CAD build for the part. Positions are in the model's coordinates, mm. A direction names the side the tool comes from. Coordinates: 2 decimals unless noted, no trailing zeros. Order: outer loops, then holes, each group sorted by start corner. A loop starts at its lowest first (then second) coordinate and runs counter-clockwise, first axis right, second up.
from build123d import *

# Parameters (mm, degrees)
F1_W      = 111.125
F1_H      = 63.0682
F2_DEPTH  = 1.5875
F3_W      = 111.125
F3_H      = 63.0682
F3_R      = 1.190625
F4_DEPTH  = 12.7
F5_R      = 2.38125
F7_DEPTH  = 1.5875
F9_R      = 1.5875
F10_DEPTH = 1.5875
F11_R     = 2.38125
F12_DEPTH = 3.175
F13_R     = 1.190625
F14_DEPTH = 4.7635
F15_R     = 1.190625
F16_DEPTH = 14.2885


with BuildPart() as f2:
    # F1 (on Top) → F2 (new body)
    with BuildSketch(Plane.XY):
        Rectangle(F1_W, F1_H)
    extrude(amount=F2_DEPTH)

    # F3 (on face) → F4 (join)
    with BuildSketch(Plane.XY.offset(1.5875)):
        Rectangle(F3_W, F3_H)
        with Locations((-53.18125, -29.15285)):
            Circle(F3_R, mode=Mode.SUBTRACT)
        with Locations((53.18125, -29.15285)):
            Circle(F3_R, mode=Mode.SUBTRACT)
        with BuildLine():
            Line((53.18125, 26.7716), (53.975, 26.7716))
            Line((53.975, 26.7716), (53.975, -26.7716))
            Line((53.975, -26.7716), (53.18125, -26.7716))
            ThreePointArc((53.18125, -26.7716), (51.497452, -27.469052), (50.8, -29.15285))
            Line((50.8, -29.15285), (50.8, -29.9466))
            Line((50.8, -29.9466), (-50.8, -29.9466))
            Line((-50.8, -29.9466), (-50.8, -29.15285))
            ThreePointArc((-50.8, -29.15285), (-51.497452, -27.469052), (-53.18125, -26.7716))
            Line((-53.18125, -26.7716), (-53.975, -26.7716))
            Line((-53.975, -26.7716), (-53.975, 26.7716))
            Line((-53.975, 26.7716), (-53.18125, 26.7716))
            ThreePointArc((-53.18125, 26.7716), (-51.497452, 27.469052), (-50.8, 29.15285))
            Line((-50.8, 29.15285), (-50.8, 29.9466))
            Line((-50.8, 29.9466), (50.8, 29.9466))
            Line((50.8, 29.9466), (50.8, 29.15285))
            ThreePointArc((50.8, 29.15285), (51.497452, 27.469052), (53.18125, 26.7716))
        make_face(mode=Mode.SUBTRACT)
        with Locations((-53.18125, 29.15285)):
            Circle(F3_R, mode=Mode.SUBTRACT)
        with Locations((53.18125, 29.15285)):
            Circle(F3_R, mode=Mode.SUBTRACT)
    extrude(amount=F4_DEPTH)

    # F5
    f5_edges = [f2.edges().sort_by_distance(p)[0] for p in [
        (55.5625, -31.5341, 7.14375),
        (55.5625, 31.5341, 7.14375),
        (-55.5625, -31.5341, 7.14375),
        (-55.5625, 31.5341, 7.14375),
    ]]
    fillet(f5_edges, radius=F5_R)

    # F6 (on face) → F7 (cut, through all)
    with BuildSketch(Plane.YZ.offset(55.5625)):
        Polygon((-13.1445, 14.2875), (-17.5895, 14.2875), (-23.4315, 14.2875), (-23.4315, 8.763), (-17.5895, 8.763), (-13.1445, 8.763), align=None)
        Polygon((5.5245, 8.763), (13.1445, 8.763), (17.5895, 8.763), (17.5895, 14.2875), (5.5245, 14.2875), align=None)
    extrude(amount=-F7_DEPTH, mode=Mode.SUBTRACT)

    # F9 (on face) → F10 (cut, through all)
    with BuildSketch(Plane(origin=(-55.5625, 0, 0), x_dir=(0, -1, 0), z_dir=(-1, 0, 0))):
        Polygon((19.05, 14.2875), (-19.05, 14.2875), (-20.955, 3.4925), (20.955, 3.4925), align=None)
        with Locations((-23.495, 8.89)):
            Circle(F9_R)
        with Locations((23.495, 8.89)):
            Circle(F9_R)
    extrude(amount=-F10_DEPTH, mode=Mode.SUBTRACT)

    # F11 (on face) → F12 (join)
    with BuildSketch(Plane.XY.offset(1.5875)):
        with Locations((0, 12.7)):
            Circle(F11_R)
        with Locations((0, -12.7)):
            Circle(F11_R)
    extrude(amount=F12_DEPTH)

    # F13 (on face) → F14 (cut, through all)
    with BuildSketch(Plane.XY.offset(4.7625)):
        with Locations((0, 12.7)):
            Circle(F13_R)
        with Locations((0, -12.7)):
            Circle(F13_R)
    extrude(amount=-F14_DEPTH, mode=Mode.SUBTRACT)

    # F15 (on face) → F16 (cut, through all)
    with BuildSketch(Plane.XY.offset(14.2875)):
        with Locations((53.18125, 29.15285)):
            Circle(F15_R)
        with Locations((53.18125, -29.15285)):
            Circle(F15_R)
        with Locations((-53.18125, -29.15285)):
            Circle(F15_R)
        with Locations((-53.18125, 29.15285)):
            Circle(F15_R)
    extrude(amount=-F16_DEPTH, mode=Mode.SUBTRACT)


solid = f2.part
1) Two-plate mould, pull along Z, no slides. Class faces 1 (the cylindrical face through (-54.78, -24.96, 8.28)), 2 (the flat face through (1, -14, 4.762)), 3 (the flat face through (-1, 0, 0)), 4 (the flat face through (-55.562, 0, 2)): released by +Z, released by -Z, zero draft, split by the parting line, or undercut.
2) Which spindle directions (+Z, -Z, +X, -X, +Y, -Y) get a long thin tool onto all of the face, cutting with end or side? Do faces 5 (the cylindrical face through (-0.31, 15.06, 3.15)), 6 (the flat face through (0, -31, 14.288)). Say none if no direction does.
3) Slice it at B-B (y = 12.7). List the corners of the cut face in (x, z) (1 decimal), plus the area to 3 significant figures.
4) Slice it at A-A (x = 0). List the corners of the cut face in (y, z).
5) Drill centre lines: probe 1 along Y at (x, z) = (0, 2.45); probe 2 along Y at (x, z) = (26, 3); probe 3 along X at (y, z) = (25, 5.75) (1 decimal). Where is each one in solid material? Low to high.
6) Slice it at C-C (y = -6). List the corners of the cut face in (x, z) (1 decimal).
7) Pin check, flat tips, straight feed: P1, Ø4, axis at x = 8.5, y = 1, coming from the +Z side; P2, Ø3, axis at x = -53.18, y = 29.15, coming from the +Z side; P3, Ø2.5, axis at x = 0, y = -12.7, coming from the +Z side; P4, Ø0.8, axis at x = 55, z = 11, coming from the +Y side. Stop position of each tip, or through.
Worked out:
1. face 1: undercut
1. face 2: released by +Z
1. face 3: released by -Z
1. face 4: zero draft
2. face 5: +Z
2. face 6: +Z, +X, -X, +Y, -Y
3. outline: (-55.6, 0) - (-1.2, 0) - (-1.2, 4.8) - (-2.4, 4.8) - (-2.4, 1.6) - (-54, 1.6) - (-54, 3.5) - (-55.6, 3.5) - close; (1.2, 0) - (55.6, 0) - (55.6, 8.8) - (54, 8.8) - (54, 1.6) - (2.4, 1.6) - (2.4, 4.8) - (1.2, 4.8) - close
3. area: 195 mm2
4. outline: (-31.53, 0) - (-13.89, 0) - (-13.89, 4.76) - (-15.08, 4.76) - (-15.08, 1.59) - (-29.95, 1.59) - (-29.95, 14.29) - (-31.53, 14.29) - close; (-11.51, 0) - (11.51, 0) - (11.51, 4.76) - (10.32, 4.76) - (10.32, 1.59) - (-10.32, 1.59) - (-10.32, 4.76) - (-11.51, 4.76) - close; (13.89, 0) - (31.53, 0) - (31.53, 14.29) - (29.95, 14.29) - (29.95, 1.59) - (15.08, 1.59) - (15.08, 4.76) - (13.89, 4.76) - close
5. probe 1: y = -31.53 to -29.95, -15.08 to -13.89, -11.51 to -10.32, 10.32 to 11.51, 13.89 to 15.08, 29.95 to 31.53
5. probe 2: y = -31.53 to -29.95, 29.95 to 31.53
5. probe 3: x = -55.6 to -54, 54 to 55.6
6. outline: (-55.6, 0) - (55.6, 0) - (55.6, 14.3) - (54, 14.3) - (54, 1.6) - (-54, 1.6) - (-54, 3.5) - (-55.6, 3.5) - close
7. P1: stops at z = 1.59
7. P2: stops at z = 14.29
7. P3: stops at z = 4.76
7. P4: stops at y = 31.07
